Source: three-view drawing plus pictorial views. Frame: mm from the lowest corner of the part. A direction names the side the tool comes from. Give positions to 0.01 mm unless a question says otherwise; leave off trailing zeros. Loops run counter-clockwise (first coordinate to the right, second up) from the corner with the lowest first, then second, coordinate; pieces in that order, holes last.
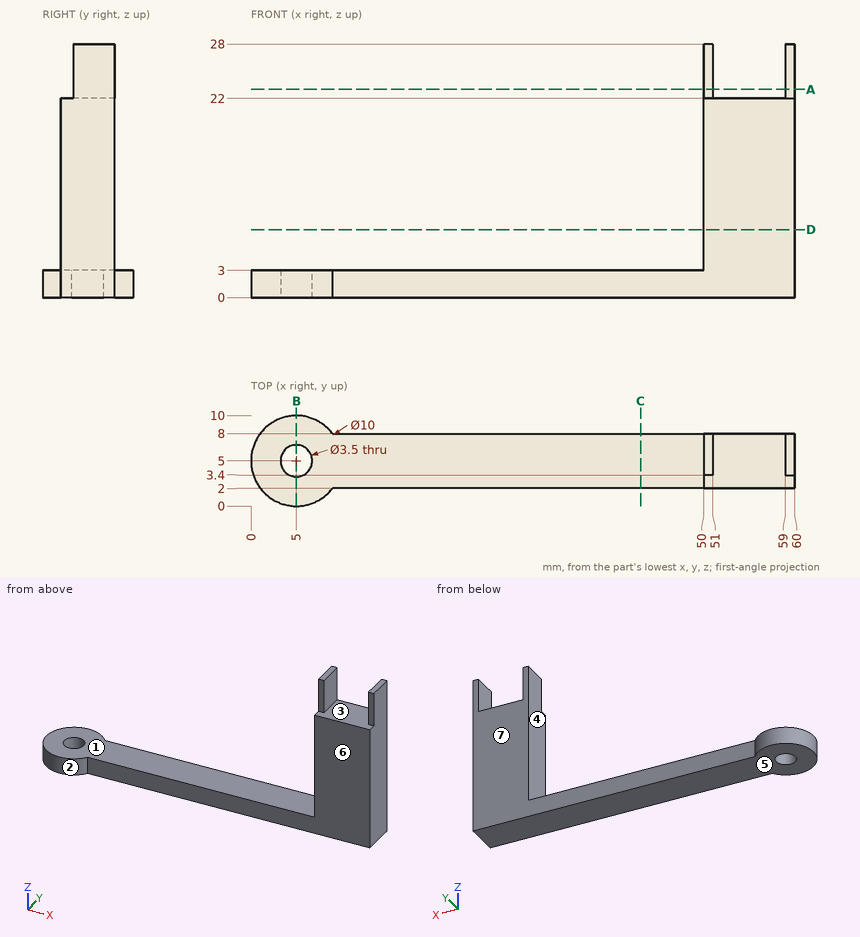
1) Cut plane A-A (z = 23). Return loops of the section in (x, y), and give its area (3 significant figures).
Checks:
outline: (50, 3.4) - (51, 3.4) - (51, 8) - (50, 8) - close; (59, 3.4) - (60, 3.4) - (60, 8) - (59, 8) - close
area: 9.20 mm2
2) Reachability of the marked faces 4, 5, 6 and 7 from +Z, -Z, +X, -X, +Y, -Y: full face, straight path, thin tool, end or side. Return the list, or none.
Checks:
face 4: +Z, -X, +Y, -Y
face 5: -Z, +X, -X, +Y, -Y
face 6: +Z, -Z, +X, -Y
face 7: +Z, -Z, +X, +Y
3) Cut plane B-B (x = 5). Return loops of the section in (y, z), and give its area (3 significant figures).
Checks:
outline: (0, 0) - (3.25, 0) - (3.25, 3) - (0, 3) - close; (6.75, 0) - (10, 0) - (10, 3) - (6.75, 3) - close
area: 19.5 mm2
4) Cut plane D-D (z = 7.5). Return loops of the section in (x, y), and give its area (3 significant figures).
Checks:
outline: (50, 2) - (60, 2) - (60, 8) - (50, 8) - close
area: 60.0 mm2
5) Ray query, probe 1 along Y at (x, z) = (5, 2.35); probe 2 along X at (y, z) = (5, 2); probe 3 along X at (y, z) = (7.75, 26.75). Return the intervals inside material, ascending.
Checks:
probe 1: y = 0 to 3.25, 6.75 to 10
probe 2: x = 0 to 3.25, 6.75 to 60
probe 3: x = 50 to 51, 59 to 60
6) Cut plane C-C (x = 43). Return loops of the section in (y, z), and give its area (3 significant figures).
Checks:
outline: (2, 0) - (8, 0) - (8, 3) - (2, 3) - close
area: 18.0 mm2
7) Pull-direction query (X, two-part tool) for the marked faces 1, 2 and 3; classes: released by +X, released by -X, zero draft, split by the parting line, or undercut.
Checks:
face 1: zero draft
face 2: split by the parting line
face 3: undercut
8) Contact query for flat-ended pins moving along their axis: P1, Ø5, axis at x = 53, y = 5, coming from the +Z side; P2, Ø3.5, axis at y = 5, z = 25.5, coming from the -X side; P3, Ø3, axis at x = 36.5, y = 8, coming from the +Z side; P4, Ø8, axis at x = 50.5, z = 15, coming from the +Y side. Output: stop coordinate, or through.
Checks:
P1: stops at z = 28
P2: stops at x = 50
P3: stops at z = 3
P4: stops at y = 8
